Read the model definition and answer for the solid it produces. Units are mm, in the model's axes. Face numbers are marked on the shaded views. Give positions to 0.01 mm unless a question says otherwise; leave off trailing zeros. Order: outer loops, then holes, each group sorted by start corner. A loop starts at its lowest first (then second) coordinate and runs counter-clockwise, first axis right, second up. Notation, with made-up numbers: (55, 7.25) -> (72, 7.25) arc R24 ccw to (72, 30.25) -> close; hole circle Ø1 at (-17.5, -9). An arc over 180 degrees is marked (long way). One line per item, written item: value. Start each with the question number.
from build123d import *

# Parameters (mm, degrees)
BOSS_EXTRUDE1_START = 22.625
SKETCH1_R           = 3.5
BOSS_EXTRUDE1_DEPTH = 0.875
BOSS_EXTRUDE2_START = 22.625
BOSS_EXTRUDE2_DEPTH = 0.875
BOSS_EXTRUDE3_START = 23.9
SKETCH3_R           = 5.05
BOSS_EXTRUDE3_DEPTH = 0.4
BOSS_EXTRUDE4_START = 23.9
SKETCH4_W           = 13.5
SKETCH4_H           = 10.207569722
BOSS_EXTRUDE4_DEPTH = 0.4
CUT_EXTRUDE1_START  = 23.025
SKETCH5_R           = 1.3
CUT_EXTRUDE1_DEPTH  = 1.275


with BuildPart() as part:
    # Sketch1 → Boss-Extrude1 (new, symmetric)
    with BuildSketch(Plane(origin=(0, 0, 0), x_dir=(1, 0, 0), z_dir=(0, 1, 0)).offset(BOSS_EXTRUDE1_START)):
        with Locations(Location((0, 0, 0), (0, 0, 270))):
            Circle(SKETCH1_R)
    extrude(amount=BOSS_EXTRUDE1_DEPTH, both=True)

    # Sketch2 → Boss-Extrude2 (add, symmetric)
    with BuildSketch(Plane(origin=(0, 0, 0), x_dir=(1, 0, 0), z_dir=(0, 1, 0)).offset(BOSS_EXTRUDE2_START)):
        Polygon((0, -3.55356197), (12.65, -2.357784906), (12.65, 2.357784906), (0, 3.55356197), align=None)
    extrude(amount=BOSS_EXTRUDE2_DEPTH, both=True)

    # Sketch3 → Boss-Extrude3 (add, symmetric)
    with BuildSketch(Plane(origin=(0, 0, 0), x_dir=(1, 0, 0), z_dir=(0, 1, 0)).offset(BOSS_EXTRUDE3_START)):
        with Locations(Location((0, 0, 0), (0, 0, 39.071364061))):
            Circle(SKETCH3_R)
    extrude(amount=BOSS_EXTRUDE3_DEPTH, both=True)

    # Sketch4 → Boss-Extrude4 (add, symmetric)
    with BuildSketch(Plane(origin=(0, 0, 0), x_dir=(1, 0, 0), z_dir=(0, 1, 0)).offset(BOSS_EXTRUDE4_START)):
        with Locations((6.75, 0)):
            Rectangle(SKETCH4_W, SKETCH4_H)
    extrude(amount=BOSS_EXTRUDE4_DEPTH, both=True)

    # Sketch5 → Cut-Extrude1 (cut, symmetric)
    with BuildSketch(Plane(origin=(0, 0, 0), x_dir=(1, 0, 0), z_dir=(0, 1, 0)).offset(CUT_EXTRUDE1_START)):
        with Locations(Location((0, 0, 0), (0, 0, 270))):
            Circle(SKETCH5_R)
    extrude(amount=CUT_EXTRUDE1_DEPTH, both=True, mode=Mode.SUBTRACT)


solid = part.part
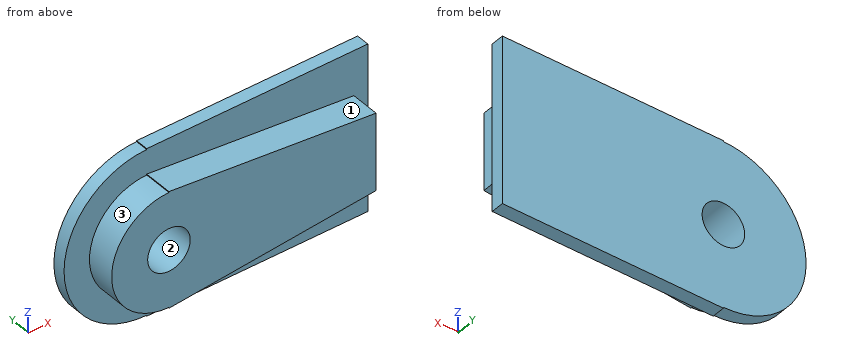
Item 1: Find section C-C on x = 1.75. Write down the section's boundary in (y, z).
Item 2: Find section D-D on z = -3. Write down the section's boundary in (x, y).
Item 3: Find section B-B on y = 24.05. Write down the section's boundary in (x, z).
Item 4: For a pull along Z with two mould halves and no side action, classify the marked faces 1, 2 and 3 as +Z half, -Z half, draft (parallel to the pull), parting line (faces both ways), or undercut.
Item 5: Find the intervals of material crossed by line 1 (X direction, y = 22.65, z = 0); line 2 (Y direction, x = 10.5, z = 4.5); line 3 (X direction, y = 23.3, z = 0.5), in increasing order. Write a range as from..to.
Item 6: Find section A-A on z = 0. Write down the section's boundary in (x, y), then the cut area to 3 significant figures.
Item 7: Flat-ended cylindrical pins translate along their axes: pin 1 (1 mm diameter, centred on y = 22.5, z = 2, fed in from -X); pin 2 (1.4 mm diameter, centred on y = 22.5, z = -0.5, fed in from +X). Find the tip coordinate at first contact, or state that the pin passes through.
Checks:
1. outline: (21.75, -3.39) -> (23.5, -3.39) -> (23.5, -5.1) -> (24.3, -5.1) -> (24.3, 5.1) -> (23.5, 5.1) -> (23.5, 3.39) -> (21.75, 3.39) -> close
2. outline: (-4.06, 23.5) -> (-1.8, 23.5) -> (-1.8, 21.75) -> (5.86, 21.75) -> (5.86, 23.5) -> (13.5, 23.5) -> (13.5, 24.3) -> (-4.06, 24.3) -> close
3. outline: (0, -5.1) -> (13.5, -5.1) -> (13.5, 5.1) -> (0, 5.1) -> (0, 5.05) arc R5.05 ccw to (0, -5.05) -> close; hole circle Ø2.6 at (0, 0)
4. face 1: +Z half
4. face 2: undercut
4. face 3: parting line
5. line 1: -3.5..-1.3, 1.3..12.65
5. line 2: 23.5..24.3
5. line 3: -3.46..-1.2, 1.2..12.65
6. outline: (-5.05, 23.5) -> (-3.5, 23.5) -> (-3.5, 21.75) -> (-1.3, 21.75) -> (-1.3, 24.3) -> (-5.05, 24.3) -> close; (1.3, 21.75) -> (12.65, 21.75) -> (12.65, 23.5) -> (13.5, 23.5) -> (13.5, 24.3) -> (1.3, 24.3) -> close
6. area: 36.5 mm2
7. pin 1: x = -3.16
7. pin 2: x = 12.65
